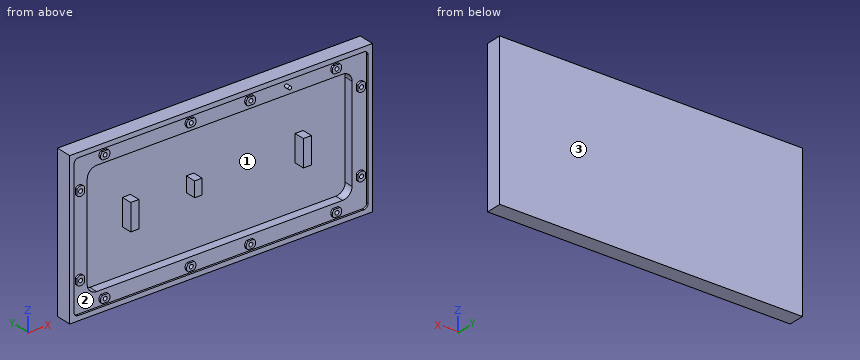
from build123d import *

# Parameters (mm, degrees)
SKETCH1_W                                  = 320
SKETCH1_H                                  = 160
BOSS_EXTRUDE1_DEPTH                        = 16.6
SKETCH1_3_W                                = 8.5
SKETCH1_3_H                                = 28
SKETCH1_3_W_2                              = 8
SKETCH1_3_H_2                              = 16
CUT_EXTRUDE1_DEPTH                         = 11.3
CUT_EXTRUDE2_DEPTH                         = 2
BOSS_EXTRUDE2_DEPTH                        = 2
SKETCH1_6_R                                = 2.1
CUT_EXTRUDE3_DEPTH                         = 6.75
MIRROR1_AT_THE_SECOND_PLANE_COPY_1_DEPTH   = 2
MIRROR1_AT_THE_SECOND_PLANE_COPY_2_SKETC_R = 2.1
MIRROR1_AT_THE_SECOND_PLANE_COPY_2_DEPTH   = 6.75
SKETCH2_R                                  = 1.65
BOSS_EXTRUDE4_DEPTH                        = 6.5
FILLET1_R                                  = 1.5


with BuildPart() as part:
    # Sketch1 → Boss-Extrude1 (new body)
    with BuildSketch(Plane(origin=(0, 0, 0), x_dir=(1, 0, 0), z_dir=(0, 1, 0))):
        Rectangle(SKETCH1_W, SKETCH1_H)
    extrude(amount=BOSS_EXTRUDE1_DEPTH)

    # Sketch1<3> → Cut-Extrude1 (cut)
    with BuildSketch(Plane(origin=(0, 0, 0), x_dir=(1, 0, 0), z_dir=(0, 1, 0))):
        with BuildLine():
            Line((130, -60), (-130, -60))
            ThreePointArc((-130, -60), (-137.071067812, -57.071067812), (-140, -50))
            Line((-140, -50), (-140, 50))
            ThreePointArc((-140, 50), (-137.071067812, 57.071067812), (-130, 60))
            Line((-130, 60), (130, 60))
            ThreePointArc((130, 60), (137.071067812, 57.071067812), (140, 50))
            Line((140, 50), (140, -50))
            ThreePointArc((140, -50), (137.071067812, -57.071067812), (130, -60))
        make_face()
        with Locations((91.25, 0)):
            Rectangle(SKETCH1_3_W, SKETCH1_3_H, mode=Mode.SUBTRACT)
        with Locations((-91.25, 0)):
            Rectangle(SKETCH1_3_W, SKETCH1_3_H, mode=Mode.SUBTRACT)
        with Locations((-24, -4)):
            Rectangle(SKETCH1_3_W_2, SKETCH1_3_H_2, mode=Mode.SUBTRACT)
    extrude(amount=CUT_EXTRUDE1_DEPTH, mode=Mode.SUBTRACT)

    # Sketch1<4> → Cut-Extrude2 (cut)
    with BuildSketch(Plane(origin=(0, 0, 0), x_dir=(1, 0, 0), z_dir=(0, 1, 0))):
        with BuildLine():
            Line((-151, -75), (151, -75))
            ThreePointArc((151, -75), (154.181980515, -73.681980515), (155.5, -70.5))
            Line((155.5, -70.5), (155.5, 70.5))
            ThreePointArc((155.5, 70.5), (154.181980515, 73.681980515), (151, 75))
            Line((151, 75), (-151, 75))
            ThreePointArc((-151, 75), (-154.181980515, 73.681980515), (-155.5, 70.5))
            Line((-155.5, 70.5), (-155.5, -70.5))
            ThreePointArc((-155.5, -70.5), (-154.181980515, -73.681980515), (-151, -75))
        make_face()
        with BuildLine():
            ThreePointArc((140, -50), (137.071067812, -57.071067812), (130, -60))
            Line((130, -60), (-130, -60))
            ThreePointArc((-130, -60), (-137.071067812, -57.071067812), (-140, -50))
            Line((-140, -50), (-140, 50))
            ThreePointArc((-140, 50), (-137.071067812, 57.071067812), (-130, 60))
            Line((-130, 60), (130, 60))
            ThreePointArc((130, 60), (137.071067812, 57.071067812), (140, 50))
            Line((140, 50), (140, -50))
        make_face(mode=Mode.SUBTRACT)
    extrude(amount=CUT_EXTRUDE2_DEPTH, mode=Mode.SUBTRACT)

    # Sketch1<5> → Boss-Extrude2 (add)
    with BuildSketch(Plane(origin=(0, 0, 0), x_dir=(1, 0, 0), z_dir=(0, 1, 0))):
        with BuildLine():
            Line((-152.5, 45.5), (-152.5, 39.5))
            ThreePointArc((-152.5, 39.5), (-148.5, 37.5), (-144.5, 39.5))
            Line((-144.5, 39.5), (-144.5, 45.5))
            ThreePointArc((-144.5, 45.5), (-148.5, 47.5), (-152.5, 45.5))
        make_face()
        with BuildLine():
            Line((-119.5, 72.3), (-125.5, 72.3))
            ThreePointArc((-125.5, 72.3), (-127.5, 68.3), (-125.5, 64.3))
            Line((-125.5, 64.3), (-119.5, 64.3))
            ThreePointArc((-119.5, 64.3), (-117.5, 68.3), (-119.5, 72.3))
        make_face()
        with BuildLine():
            Line((-34.5, 72.3), (-28.5, 72.3))
            ThreePointArc((-28.5, 72.3), (-26.5, 68.3), (-28.5, 64.3))
            Line((-28.5, 64.3), (-34.5, 64.3))
            ThreePointArc((-34.5, 64.3), (-36.5, 68.3), (-34.5, 72.3))
        make_face()
    boss_extrude2 = extrude(amount=BOSS_EXTRUDE2_DEPTH)

    # Sketch1<6> → Cut-Extrude3 (cut)
    with BuildSketch(Plane(origin=(0, 0, 0), x_dir=(1, 0, 0), z_dir=(0, 1, 0))):
        with Locations(Location((-148.5, 42.5, 0), (0, 0, 270))):
            Circle(SKETCH1_6_R)
        with Locations(Location((-122.5, 68.3, 0), (0, 0, 270))):
            Circle(SKETCH1_6_R)
        with Locations(Location((-31.5, 68.3, 0), (0, 0, 270))):
            Circle(SKETCH1_6_R)
    cut_extrude3 = extrude(amount=CUT_EXTRUDE3_DEPTH, mode=Mode.SUBTRACT)

    # Mirror1: Boss-Extrude2, Cut-Extrude3 across plane
    add(boss_extrude2.mirror(Plane.XY))
    add(cut_extrude3.mirror(Plane.XY), mode=Mode.SUBTRACT)

    # Mirror1 at the second plane: Boss-Extrude2, Cut-Extrude3 across plane
    add(boss_extrude2.mirror(Plane(origin=(0, 0, 0), x_dir=(0, 0, 1), z_dir=(1, 0, 0))))
    add(cut_extrude3.mirror(Plane(origin=(0, 0, 0), x_dir=(0, 0, 1), z_dir=(1, 0, 0))), mode=Mode.SUBTRACT)

    # Mirror1 at the second plane copy 1 sketc → Mirror1 at the second plane copy 1 (add)
    with BuildSketch(Plane(origin=(0, 0, 0), x_dir=(-1, 0, 0), z_dir=(0, 1, 0))):
        with BuildLine():
            Line((-152.5, 45.5), (-152.5, 39.5))
            ThreePointArc((-152.5, 39.5), (-148.5, 37.5), (-144.5, 39.5))
            Line((-144.5, 39.5), (-144.5, 45.5))
            ThreePointArc((-144.5, 45.5), (-148.5, 47.5), (-152.5, 45.5))
        make_face()
        with BuildLine():
            Line((-119.5, 72.3), (-125.5, 72.3))
            ThreePointArc((-125.5, 72.3), (-127.5, 68.3), (-125.5, 64.3))
            Line((-125.5, 64.3), (-119.5, 64.3))
            ThreePointArc((-119.5, 64.3), (-117.5, 68.3), (-119.5, 72.3))
        make_face()
        with BuildLine():
            Line((-34.5, 72.3), (-28.5, 72.3))
            ThreePointArc((-28.5, 72.3), (-26.5, 68.3), (-28.5, 64.3))
            Line((-28.5, 64.3), (-34.5, 64.3))
            ThreePointArc((-34.5, 64.3), (-36.5, 68.3), (-34.5, 72.3))
        make_face()
    extrude(amount=MIRROR1_AT_THE_SECOND_PLANE_COPY_1_DEPTH)

    # Mirror1 at the second plane copy 2 sketc → Mirror1 at the second plane copy 2 (cut)
    with BuildSketch(Plane(origin=(0, 0, 0), x_dir=(-1, 0, 0), z_dir=(0, 1, 0))):
        with Locations(Location((-148.5, 42.5, 0), (0, 0, 270))):
            Circle(MIRROR1_AT_THE_SECOND_PLANE_COPY_2_SKETC_R)
        with Locations(Location((-122.5, 68.3, 0), (0, 0, 270))):
            Circle(MIRROR1_AT_THE_SECOND_PLANE_COPY_2_SKETC_R)
        with Locations(Location((-31.5, 68.3, 0), (0, 0, 270))):
            Circle(MIRROR1_AT_THE_SECOND_PLANE_COPY_2_SKETC_R)
    extrude(amount=MIRROR1_AT_THE_SECOND_PLANE_COPY_2_DEPTH, mode=Mode.SUBTRACT)

    # Sketch2 → Boss-Extrude4 (add)
    with BuildSketch(Plane.XZ.offset(-2)):
        with Locations(Location((70.2, 69, 0), (0, 0, 90))):
            Circle(SKETCH2_R)
    extrude(amount=BOSS_EXTRUDE4_DEPTH)

    # Fillet1
    fillet1_edges = [part.edges().sort_by_distance(p)[0] for p in [
        (70.2, -4.5, 67.35),
    ]]
    fillet(fillet1_edges, radius=FILLET1_R)


solid = part.part
The listing builds one solid part. Answer for the finished solid, in the listing's coordinates (mm). Face numbers are marked on the shaded views. Round coordinates to 2 decimals unless told otherwise and drop trailing zeros. Order: outer loops, then holes, each group sorted by start corner. A loop starts at its lowest first (then second) coordinate and runs counter-clockwise, first axis right, second up. Notation, with made-up numbers: (3, -18.75) -> (45, -18.75) arc R16 ccw to (45, 7.25) -> close; hole circle Ø7 at (1, -33). An arc over 180 degrees is marked (long way). Put each result on its own line as item: value.
Q1. Consider line 1 along X through (y, z) = (4, 68.3); line 2 along Z through (x, y) = (31.5, 2.25); line 3 along Z through (x, y) = (-27.5, 7.5). Determine where each line is inside the solid, lowest interval first.
Results list:
line 1: -160 to -124.6, -120.4 to -33.6, -29.4 to 29.4, 33.6 to 120.4, 124.6 to 160
line 2: -80 to -70.4, -66.2 to -60, 60 to 66.2, 70.4 to 80
line 3: -80 to -60, -4 to 12, 60 to 80
Q2. Determine the mould class of the marked faces 1, 2 and 3 for opening direction Z: pulls with the +Z half, pulls with the -Z half, needs draft (parallel to the pull), parting line crosses it, or undercut.
Results list:
face 1: undercut
face 2: undercut
face 3: needs draft
Q3. Section B-B, the plane z = -33.5 is taken. Write down the section's boundary in (x, y).
Results list:
outline: (-160, 0) -> (-155.5, 0) -> (-155.5, 2) -> (-140, 2) -> (-140, 11.3) -> (140, 11.3) -> (140, 2) -> (155.5, 2) -> (155.5, 0) -> (160, 0) -> (160, 16.6) -> (-160, 16.6) -> close
Q4. Section A-A, the plane x = 44.5 is taken. Write down the section's boundary in (y, z).
Results list:
outline: (0, -80) -> (16.6, -80) -> (16.6, 80) -> (0, 80) -> (0, 75) -> (2, 75) -> (2, 60) -> (11.3, 60) -> (11.3, -60) -> (2, -60) -> (2, -75) -> (0, -75) -> close
Q5. Each of these flat-tipped pins is pushed along its axis until it touches: P1, Ø1.3, axis at x = -149, z = -42.5, coming from the -Y side; P2, Ø6, axis at x = -17.5, z = 63, coming from the -Y side; P3, Ø9, axis at x = -122.5, z = -66.5, coming from the -Y side. Where does it stop, or does it pass through?
Results list:
P1: y = 6.75
P2: y = 2
P3: y = 0
